The listing builds one solid part. Answer for the finished solid, in the listing's coordinates (mm). Face numbers are marked on the shaded views. A direction names the side the tool comes from. Coordinates: 2 decimals unless noted, no trailing zeros. Loops run counter-clockwise (first coordinate to the right, second up) from the corner with the lowest first, then second, coordinate; pieces in that order, holes last. Notation, with made-up numbers: M 50.25,11 L 99.25,11 A27 cw 99.25,44 Z; hole C -2.5,-3.75 d4. An arc over 180 degrees is marked long. Return JSON: item names as keys, results as strings. Group by question number.
1. Straight lines are drawn through the part: L1, parallel to Y at x = -6.25, z = 0; L2, parallel to X at y = -36, z = -16.5; L3, parallel to Y at x = -19, z = -18. For each, find the intervals that lie inside material, in ascending order. Write a range as from..to.
2. Section A-A (z = 0) is taken. Write down the section's boundary in (x, y), then the cut area to 3 significant figures.
3. The mould has two halves that part along Z. Classify the marked faces 1, 2 and 3: pulls with the +Z half, pulls with the -Z half, needs draft (parallel to the pull), parting line crosses it, or undercut.
4. Section C-C (z = 32.5) is taken. Write down the section's boundary in (x, y), then the cut area to 3 significant figures.
5. Section B-B (y = -35) is taken. Write down the section's boundary in (x, z).
6. Section D-D (x = -8.75) is taken. Write down the section's boundary in (y, z), then the cut area to 3 significant figures.
7. Given P1, Ø2, axis at x = -15, y = -14.5, coming from the -Z side; P2, Ø2, axis at x = -16.5, y = 34.5, coming from the -Z side; P3, Ø13, axis at y = -35, z = 0, coming from the -X side; P4, Ø8, axis at x = -6, y = 5, coming from the -Z side, each flat-ended and moving along its own axis, determine where each tip first touches the part or whether it passes through.
8. Which of the six approach directions +Z, -Z, +X, -X, +Y, -Y give full straight-line access (tool end or side, diameter ignored) to the marked faces 4 and 5?
```python
from build123d import *

# Parameters (mm, degrees)
SKETCH2_R          = 4
CUT_EXTRUDE1_DEPTH = 65.776538963


with BuildPart() as part:
    # Sketch1 → Revolve1 (revolve)
    with BuildSketch(Plane.XY, mode=Mode.PRIVATE) as revolve1_sk:
        Polygon((-13.637426901, 11), (-3.637426901, 11), (-3.637426901, 44), (-13.637426901, 44), (-13.637426901, 26), (-21.637426901, 26), (-21.637426901, 22), (-13.637426901, 22), align=None)
    revolve(revolve1_sk.sketch.rotate(Axis((-28.771929825, 0, 0), (1, 0, 0)), 90), axis=Axis((-28.771929825, 0, 0), (1, 0, 0)))

    # Sketch2 → Cut-Extrude1 (cut, through all)
    with BuildSketch(Plane(origin=(-3.637426901, 0, 0), x_dir=(0, 0, -1), z_dir=(1, 0, 0))):
        with Locations((0, 35)):
            Circle(SKETCH2_R)
        with Locations((35, 0)):
            Circle(SKETCH2_R)
        with Locations((0, -35)):
            Circle(SKETCH2_R)
        with Locations((-35, 0)):
            Circle(SKETCH2_R)
    extrude(amount=-CUT_EXTRUDE1_DEPTH, mode=Mode.SUBTRACT)


solid = part.part
```
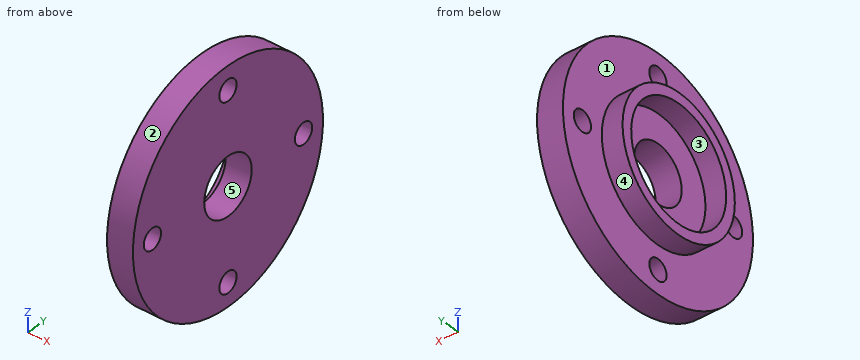
Worked out:
{
 "1": {"L1": "-44..-39, -31..-11, 11..31, 39..44", "L2": "-13.64..-3.64", "L3": "-18.76..-12.65, 12.65..18.76"},
 "2": {"outline": "M -21.64,-26 L -13.64,-26 L -13.64,-31 L -3.64,-31 L -3.64,-11 L -13.64,-11 L -13.64,-22 L -21.64,-22 Z; M -21.64,22 L -13.64,22 L -13.64,11 L -3.64,11 L -3.64,31 L -13.64,31 L -13.64,26 L -21.64,26 Z; M -13.64,-44 L -3.64,-44 L -3.64,-39 L -13.64,-39 Z; M -13.64,39 L -3.64,39 L -3.64,44 L -13.64,44 Z", "area": "564 mm^2"},
 "3": {"face 1": "needs draft", "face 2": "parting line crosses it", "face 3": "undercut"},
 "4": {"outline": "M -13.64,-29.66 L -3.64,-29.66 L -3.64,-3.12 L -13.64,-3.12 Z; M -13.64,3.12 L -3.64,3.12 L -3.64,29.66 L -13.64,29.66 Z", "area": "531 mm^2"},
 "5": {"outline": "M -13.64,-26.66 L -3.64,-26.66 L -3.64,-4 L -13.64,-4 Z; M -13.64,4 L -3.64,4 L -3.64,26.66 L -13.64,26.66 Z"},
 "6": {"outline": "C 0,0 d88; hole C -35,0 d8; hole C 0,0 d22; hole C 0,-35 d8; hole C 0,35 d8; hole C 35,0 d8", "area": "5,500 mm^2"},
 "7": {"P1": "z = -22.22", "P2": "through", "P3": "x = -13.64", "P4": "z = -43.99"},
 "8": {"face 4": "-X", "face 5": "+X, -X"}
}
